from build123d import *

# Parameters (mm, degrees)
REVOLVE1_OUTLINE_R     = 2.5
REVOLVE1_DEPTH         = 21
REVOLVE1_2_OUTLINE_R   = 4.25
REVOLVE1_2_OUTLINE_R_2 = 2.5
REVOLVE1_2_DEPTH       = 5
FILLET1_R              = 0.1
FILLET2_R              = 0.12
CHAMFER1_SIZE          = 0.2
EXTRUDE1_DEPTH         = 3.5


# Read off the part's stored shape, not the designer's step: Revolve1
with BuildPart() as part:
    # Revolve1 outline → Revolve1 (new body)
    with BuildSketch(Plane.YZ):
        Circle(REVOLVE1_OUTLINE_R)
    extrude(amount=REVOLVE1_DEPTH)

    # Revolve1 2 outline → Revolve1 2 (add)
    with BuildSketch(Plane.YZ):
        Circle(REVOLVE1_2_OUTLINE_R)
        Circle(REVOLVE1_2_OUTLINE_R_2, mode=Mode.SUBTRACT)
    extrude(amount=REVOLVE1_2_DEPTH)

    # Fillet1
    fillet1_edges = [part.edges().sort_by_distance(p)[0] for p in [
        (5, -2.5, 0),
    ]]
    fillet(fillet1_edges, radius=FILLET1_R)

    # Fillet2
    fillet2_edges = [part.edges().sort_by_distance(p)[0] for p in [
        (0, -4.25, 0),
    ]]
    fillet(fillet2_edges, radius=FILLET2_R)

    # Chamfer1
    chamfer1_edges = [part.edges().sort_by_distance(p)[0] for p in [
        (21, -2.5, 0),
    ]]
    chamfer(chamfer1_edges, length=CHAMFER1_SIZE)

    # Sketch2 → Extrude1 (cut)
    with BuildSketch(Plane.ZY):
        Polygon((0, 2.309401077), (-2, 1.154700538), (-2, -1.154700538), (0, -2.309401077), (2, -1.154700538), (2, 1.154700538), align=None)
    extrude(amount=-EXTRUDE1_DEPTH, mode=Mode.SUBTRACT)


solid = part.part
Geometry: final body of the model. Coordinates: model frame, mm. A direction names the side the tool comes from. Give positions to 0.01 mm unless a question says otherwise; leave off trailing zeros. Order: outer loops, then holes, each group sorted by start corner. A loop starts at its lowest first (then second) coordinate and runs counter-clockwise, first axis right, second up. Notation, with made-up numbers: (12, 62.25) -> (61, 62.25) arc R15 ccw to (61, 71.25) -> close; hole circle Ø5 at (67.25, 60.5). An arc over 180 degrees is marked (long way). Answer as a JSON object with one key per item and string values.
Q1. First-contact query: pin 1 (5 mm diameter, centred on x = 12, z = 0, fed in from +Y); pin 2 (1 mm diameter, centred on x = 8.5, z = -1.5, fed in from +Y); pin 3 (0.7 mm diameter, centred on x = 2.5, y = 0.5, fed in from -Z). Flat tips, straight axial feed; report the tip coordinate or a pass-through.
Entries:
{"pin 1": "stops at y = 2.5", "pin 2": "stops at y = 2.29", "pin 3": "stops at z = -4.25"}
Q2. Draft query along Y for faces 1 (the cylindrical face through (2.526, 2.285, 3.584)), 2 (the flat face through (0, 2, 1)), 3 (the flat face through (1.73, 1.74, -0.99)). Return one class per face: released by +Y, released by -Y, zero draft, split by the parting line, or undercut.
Entries:
{"face 1": "split by the parting line", "face 2": "zero draft", "face 3": "undercut"}
Q3. Section A-A (y = 0). Output: boundary loops of the cut face in (x, z), plus the area to 3 significant figures.
Entries:
{"outline": "(0, -4.13) arc R0.12 ccw to (0.12, -4.25) -> (5, -4.25) -> (5, -2.6) arc R0.1 cw to (5.1, -2.5) -> (20.8, -2.5) -> (21, -2.3) -> (21, 2.3) -> (20.8, 2.5) -> (5.1, 2.5) arc R0.1 cw to (5, 2.6) -> (5, 4.25) -> (0.12, 4.25) arc R0.12 ccw to (0, 4.13) -> (0, 2) -> (3.5, 2) -> (3.5, -2) -> (0, -2) -> close", "area": "108 mm^2"}
Q4. Material intervals for probe 1 along X at (y, z) = (-1, 0.5); probe 2 along Y at (x, z) = (1.25, -0.25); probe 3 along X at (y, z) = (-1.25, -3.5), sorted ascending.
Entries:
{"probe 1": "x = 3.5 to 21", "probe 2": "y = -4.24 to -2.17, 2.17 to 4.24", "probe 3": "x = 0 to 5"}
Q5. Section B-B (x = 11.75). Output: boundary loops of the cut face in (y, z).
Entries:
{"outline": "circle Ø5 at (0, 0)"}
Q6. Access query for faces 4 (the flat face through (1.73, -1.74, 0.99)), 5 (the cylindrical face through (12.84, -0.54, -2.44)), 6 (the flat face through (21, 0, 0)). Directions: +Z, -Z, +X, -X, +Y, -Y. A direction counts if a zero-diameter tool reaches every point of the face in a straight line with its end or side. Return the directions, or none.
Entries:
{"face 4": "-X", "face 5": "+X", "face 6": "+Z, -Z, +X, +Y, -Y"}
